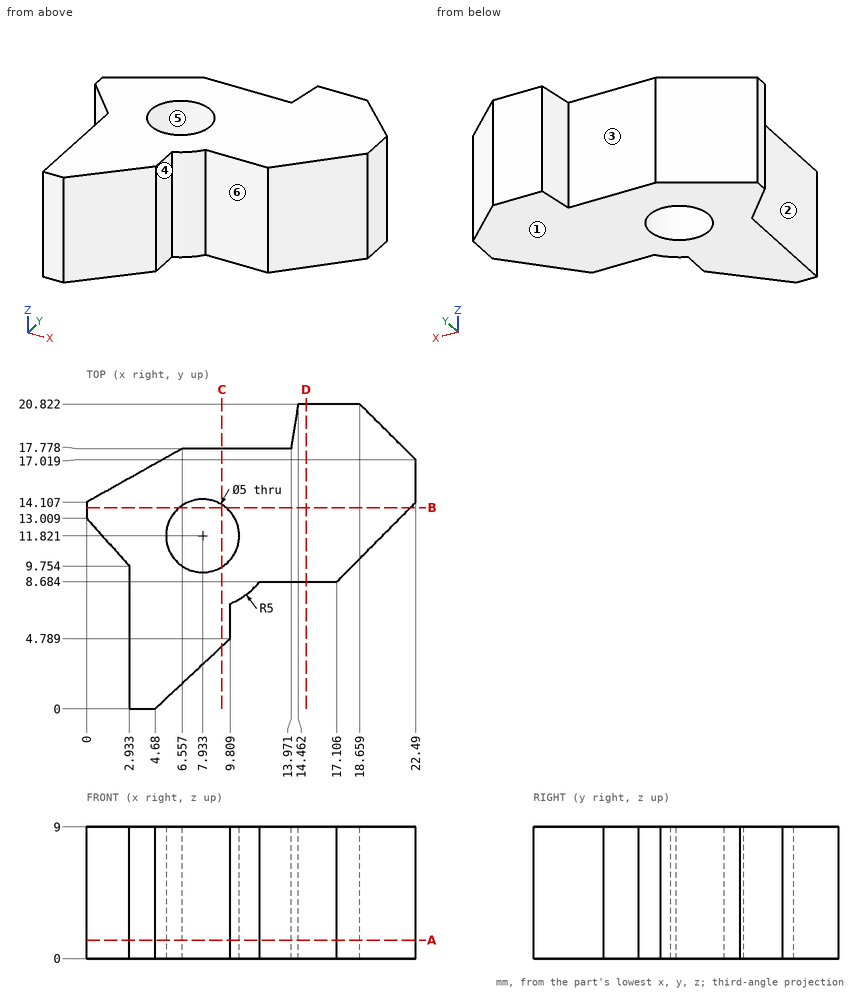
Answer from the drawing. Dimensions are ordinates in mm from the lowest x, y and z of the part. A direction names the side the tool comes from. Coordinates: 2 decimals unless noted, no trailing zeros. Loops run counter-clockwise (first coordinate to the right, second up) from the corner with the lowest first, then second, coordinate; pieces in that order, holes last. Notation, with made-up numbers: (20, 34) -> (36, 34) arc R23 ccw to (36, 73) -> close; hole circle Ø3 at (22.5, 66). An arc over 180 degrees is marked (long way). Answer as CSV lines item,"result".
Q1. The part is cut by section B-B on y = 13.75. Write down the section's boundary in (x, z) (1 decimal).
Findings:
outline,"(0, 0) -> (6.3, 0) -> (6.3, 9) -> (0, 9) -> close; (9.5, 0) -> (22.1, 0) -> (22.1, 9) -> (9.5, 9) -> close"
Q2. A tool of negligible diameter and unlimited length cuts with its end or side. For the marked faces 1, 2 and 3, from which of +Z, -Z, +X, -X, +Y, -Y can it reach the whole face along a straight path? Write none if from no direction.
Findings:
face 1,"-Z, +X, -X, +Y, -Y"
face 2,"+Z, -Z, -X, -Y"
face 3,"+Z, -Z, -X, +Y"
Q3. The part is cut by section A-A on z = 1.25. Write down the section's boundary in (x, y) (1 decimal).
Findings:
outline,"(0, 13) -> (2.9, 9.8) -> (2.9, 0) -> (4.7, 0) -> (9.8, 4.8) -> (9.8, 7.2) arc R5 ccw to (11.8, 8.7) -> (17.1, 8.7) -> (22.5, 14.1) -> (22.5, 17) -> (18.7, 20.8) -> (14.5, 20.8) -> (14, 17.8) -> (6.6, 17.8) -> (0, 14.1) -> close; hole circle Ø5 at (7.9, 11.8)"
Q4. The part is cut by section C-C on x = 9.25. Write down the section's boundary in (y, z) (1 decimal).
Findings:
outline,"(4.3, 0) -> (9.7, 0) -> (9.7, 9) -> (4.3, 9) -> close; (13.9, 0) -> (17.8, 0) -> (17.8, 9) -> (13.9, 9) -> close"
Q5. The part is cut by section D-D on x = 15. Write down the section's boundary in (y, z).
Findings:
outline,"(8.68, 0) -> (20.82, 0) -> (20.82, 9) -> (8.68, 9) -> close"
Q6. For a pull along Y with two mould halves and no side action, classify the marked faces 4, 5 and 6 as +Y half, -Y half, draft (parallel to the pull), parting line (faces both ways), or undercut.
Findings:
face 4,"draft"
face 5,"undercut"
face 6,"-Y half"
Q7. Each of these flat-tipped pins is pushed along its axis until it touches: pin 1 (3 mm diameter, centred on x = 3, z = 3.5, fed in from +Y); pin 2 (1.5 mm diameter, centred on y = 5, z = 6, fed in from -X); pin 3 (2.5 mm diameter, centred on x = 14, z = 5, fed in from -Y). Where does it stop, or does it pass through?
Findings:
pin 1,"stops at y = 16.63"
pin 2,"stops at x = 2.93"
pin 3,"stops at y = 8.68"
Q8. Find the intervals of material crossed by probe 1 along Y at (x, z) = (5.75, 3) (1 decimal); probe 2 along Y at (x, z) = (15.75, 3.5); probe 3 along Y at (x, z) = (13.25, 2), in increasing order.
Findings:
probe 1,"y = 1 to 10.6, 13 to 17.3"
probe 2,"y = 8.68 to 20.82"
probe 3,"y = 8.68 to 17.78"
